```python
from build123d import *

# Parameters (mm, degrees)
BOSS_EXTRUDE1_DEPTH          = 6
FILLET1_R                    = 20
SKETCH2_R                    = 1.7
CUT_EXTRUDE1_DEPTH           = 133.106886392
CIRPATTERN1_COUNT            = 4
SKETCH3_R                    = 1.6
CUT_EXTRUDE2_DEPTH           = 133.106886392
LPATTERN1_COUNT              = 6
LPATTERN1_PITCH              = 10
CIRPATTERN2_COUNT            = 4
CIRPATTERN2_COPY_1_SKETCH_R  = 1.6
CIRPATTERN2_COPY_1_DEPTH     = 133.106886392
CIRPATTERN2_COPY_2_SKETCH_R  = 1.6
CIRPATTERN2_COPY_2_DEPTH     = 133.106886392
CIRPATTERN2_COPY_3_SKETCH_R  = 1.6
CIRPATTERN2_COPY_3_DEPTH     = 133.106886392
CIRPATTERN2_COPY_4_SKETCH_R  = 1.6
CIRPATTERN2_COPY_4_DEPTH     = 133.106886392
CIRPATTERN2_COPY_5_SKETCH_R  = 1.6
CIRPATTERN2_COPY_5_DEPTH     = 133.106886392
CIRPATTERN2_COPY_6_SKETCH_R  = 1.6
CIRPATTERN2_COPY_6_DEPTH     = 133.106886392
CIRPATTERN2_COPY_7_SKETCH_R  = 1.6
CIRPATTERN2_COPY_7_DEPTH     = 133.106886392
CIRPATTERN2_COPY_8_SKETCH_R  = 1.6
CIRPATTERN2_COPY_8_DEPTH     = 133.106886392
CIRPATTERN2_COPY_9_SKETCH_R  = 1.6
CIRPATTERN2_COPY_9_DEPTH     = 133.106886392
CIRPATTERN2_COPY_10_SKETCH_R = 1.6
CIRPATTERN2_COPY_10_DEPTH    = 133.106886392
CIRPATTERN2_COPY_11_SKETCH_R = 1.6
CIRPATTERN2_COPY_11_DEPTH    = 133.106886392
CIRPATTERN2_COPY_12_SKETCH_R = 1.6
CIRPATTERN2_COPY_12_DEPTH    = 133.106886392
CIRPATTERN2_COPY_13_SKETCH_R = 1.6
CIRPATTERN2_COPY_13_DEPTH    = 133.106886392
CIRPATTERN2_COPY_14_SKETCH_R = 1.6
CIRPATTERN2_COPY_14_DEPTH    = 133.106886392
CIRPATTERN2_COPY_15_SKETCH_R = 1.6
CIRPATTERN2_COPY_15_DEPTH    = 133.106886392
SKETCH4_R                    = 1.7
CUT_EXTRUDE3_DEPTH           = 133.106886392
CIRPATTERN3_COUNT            = 4
SKETCH5_R                    = 1.7
CUT_EXTRUDE4_DEPTH           = 133.106886392
SKETCH7_R                    = 1.7
CUT_EXTRUDE5_DEPTH           = 133.106886392
LPATTERN2_COUNT              = 2
LPATTERN2_PITCH              = 10
LPATTERN2_COL_COUNT          = 2
LPATTERN2_COL_PITCH          = 10
MIRROR2_COPY_1_SKETCH_R      = 1.7
MIRROR2_COPY_1_DEPTH         = 133.106886392
MIRROR2_COPY_2_SKETCH_R      = 1.7
MIRROR2_COPY_2_DEPTH         = 133.106886392


with BuildPart() as part:
    # Sketch1 → Boss-Extrude1 (new body)
    with BuildSketch(Plane(origin=(0, 0, 0), x_dir=(1, 0, 0), z_dir=(0, 1, 0))):
        with BuildLine():
            Line((-72.831998462, 89.802561211), (-13.029437252, 30))
            Line((-13.029437252, 30), (13.029437252, 30))
            Line((13.029437252, 30), (72.831998462, 89.802561211))
            ThreePointArc((72.831998462, 89.802561211), (89.802561211, 89.802561211), (89.802561211, 72.831998462))
            Line((89.802561211, 72.831998462), (30, 13.029437252))
            Line((30, 13.029437252), (30, -13.029437252))
            Line((30, -13.029437252), (89.802561211, -72.831998462))
            ThreePointArc((89.802561211, -72.831998462), (89.802561211, -89.802561211), (72.831998462, -89.802561211))
            Line((72.831998462, -89.802561211), (13.029437252, -30))
            Line((13.029437252, -30), (-13.029437252, -30))
            Line((-13.029437252, -30), (-72.831998462, -89.802561211))
            ThreePointArc((-72.831998462, -89.802561211), (-89.802561211, -89.802561211), (-89.802561211, -72.831998462))
            Line((-89.802561211, -72.831998462), (-30, -13.029437252))
            Line((-30, -13.029437252), (-30, 13.029437252))
            Line((-30, 13.029437252), (-89.802561211, 72.831998462))
            ThreePointArc((-89.802561211, 72.831998462), (-89.802561211, 89.802561211), (-72.831998462, 89.802561211))
        make_face()
    extrude(amount=BOSS_EXTRUDE1_DEPTH)

    # Fillet1
    fillet1_edges = [part.edges().sort_by_distance(p)[0] for p in [
        (-13.029437252, 3, -30),
        (13.029437252, 3, -30),
        (30, 3, -13.029437252),
        (30, 3, 13.029437252),
        (13.029437252, 3, 30),
        (-13.029437252, 3, 30),
        (-30, 3, 13.029437252),
        (-30, 3, -13.029437252),
    ]]
    fillet(fillet1_edges, radius=FILLET1_R)

    # Sketch2 → Cut-Extrude1 (cut, through all)
    with BuildSketch(Plane(origin=(0, 6, 0), x_dir=(1, 0, 0), z_dir=(0, 1, 0))):
        with Locations(Location((-22.525, -22.525, 0), (0, 0, 270))):
            Circle(SKETCH2_R)
    cut_extrude1 = extrude(amount=-CUT_EXTRUDE1_DEPTH, mode=Mode.SUBTRACT)

    # CirPattern1: Cut-Extrude1 ×4 about axis
    cirpattern1_axis = Axis((0, 0, 0), (0, 1, 0))
    for i in range(1, CIRPATTERN1_COUNT):
        add(cut_extrude1.rotate(cirpattern1_axis, i * 360 / CIRPATTERN1_COUNT), mode=Mode.SUBTRACT)

    # Sketch3 → Cut-Extrude2 (cut, through all)
    with BuildSketch(Plane(origin=(0, 6, 0), x_dir=(1, 0, 0), z_dir=(0, 1, 0))):
        with Locations(Location((-30, -30, 0), (0, 0, 270))):
            Circle(SKETCH3_R)
    cut_extrude2 = extrude(amount=-CUT_EXTRUDE2_DEPTH, mode=Mode.SUBTRACT)

    # LPattern1: Cut-Extrude2 ×6
    with Locations(*[Vector(-0.7071067811865467, 0, 0.7071067811865485) * (i * LPATTERN1_PITCH) for i in range(1, LPATTERN1_COUNT)]):
        add(cut_extrude2, mode=Mode.SUBTRACT)

    # CirPattern2: Cut-Extrude2 ×4 about axis
    cirpattern2_axis = Axis((0, 6.3, 0), (0, -1, 0))
    for i in range(1, CIRPATTERN2_COUNT):
        add(cut_extrude2.rotate(cirpattern2_axis, i * 360 / CIRPATTERN2_COUNT), mode=Mode.SUBTRACT)

    # CirPattern2 copy 1 sketch → CirPattern2 copy 1 (cut, through all)
    with BuildSketch(Plane(origin=(-7.071067812, 6, -7.071067812), x_dir=(0, 0, 1), z_dir=(0, 1, 0))):
        with Locations(Location((-30, -30, 0), (0, 0, 270))):
            Circle(CIRPATTERN2_COPY_1_SKETCH_R)
    extrude(amount=-CIRPATTERN2_COPY_1_DEPTH, mode=Mode.SUBTRACT)

    # CirPattern2 copy 2 sketch → CirPattern2 copy 2 (cut, through all)
    with BuildSketch(Plane(origin=(7.071067812, 6, -7.071067812), x_dir=(-1, 0, 0), z_dir=(0, 1, 0))):
        with Locations(Location((-30, -30, 0), (0, 0, 270))):
            Circle(CIRPATTERN2_COPY_2_SKETCH_R)
    extrude(amount=-CIRPATTERN2_COPY_2_DEPTH, mode=Mode.SUBTRACT)

    # CirPattern2 copy 3 sketch → CirPattern2 copy 3 (cut, through all)
    with BuildSketch(Plane(origin=(7.071067812, 6, 7.071067812), x_dir=(0, 0, -1), z_dir=(0, 1, 0))):
        with Locations(Location((-30, -30, 0), (0, 0, 270))):
            Circle(CIRPATTERN2_COPY_3_SKETCH_R)
    extrude(amount=-CIRPATTERN2_COPY_3_DEPTH, mode=Mode.SUBTRACT)

    # CirPattern2 copy 4 sketch → CirPattern2 copy 4 (cut, through all)
    with BuildSketch(Plane(origin=(-14.142135624, 6, -14.142135624), x_dir=(0, 0, 1), z_dir=(0, 1, 0))):
        with Locations(Location((-30, -30, 0), (0, 0, 270))):
            Circle(CIRPATTERN2_COPY_4_SKETCH_R)
    extrude(amount=-CIRPATTERN2_COPY_4_DEPTH, mode=Mode.SUBTRACT)

    # CirPattern2 copy 5 sketch → CirPattern2 copy 5 (cut, through all)
    with BuildSketch(Plane(origin=(14.142135624, 6, -14.142135624), x_dir=(-1, 0, 0), z_dir=(0, 1, 0))):
        with Locations(Location((-30, -30, 0), (0, 0, 270))):
            Circle(CIRPATTERN2_COPY_5_SKETCH_R)
    extrude(amount=-CIRPATTERN2_COPY_5_DEPTH, mode=Mode.SUBTRACT)

    # CirPattern2 copy 6 sketch → CirPattern2 copy 6 (cut, through all)
    with BuildSketch(Plane(origin=(14.142135624, 6, 14.142135624), x_dir=(0, 0, -1), z_dir=(0, 1, 0))):
        with Locations(Location((-30, -30, 0), (0, 0, 270))):
            Circle(CIRPATTERN2_COPY_6_SKETCH_R)
    extrude(amount=-CIRPATTERN2_COPY_6_DEPTH, mode=Mode.SUBTRACT)

    # CirPattern2 copy 7 sketch → CirPattern2 copy 7 (cut, through all)
    with BuildSketch(Plane(origin=(-21.213203436, 6, -21.213203436), x_dir=(0, 0, 1), z_dir=(0, 1, 0))):
        with Locations(Location((-30, -30, 0), (0, 0, 270))):
            Circle(CIRPATTERN2_COPY_7_SKETCH_R)
    extrude(amount=-CIRPATTERN2_COPY_7_DEPTH, mode=Mode.SUBTRACT)

    # CirPattern2 copy 8 sketch → CirPattern2 copy 8 (cut, through all)
    with BuildSketch(Plane(origin=(21.213203436, 6, -21.213203436), x_dir=(-1, 0, 0), z_dir=(0, 1, 0))):
        with Locations(Location((-30, -30, 0), (0, 0, 270))):
            Circle(CIRPATTERN2_COPY_8_SKETCH_R)
    extrude(amount=-CIRPATTERN2_COPY_8_DEPTH, mode=Mode.SUBTRACT)

    # CirPattern2 copy 9 sketch → CirPattern2 copy 9 (cut, through all)
    with BuildSketch(Plane(origin=(21.213203436, 6, 21.213203436), x_dir=(0, 0, -1), z_dir=(0, 1, 0))):
        with Locations(Location((-30, -30, 0), (0, 0, 270))):
            Circle(CIRPATTERN2_COPY_9_SKETCH_R)
    extrude(amount=-CIRPATTERN2_COPY_9_DEPTH, mode=Mode.SUBTRACT)

    # CirPattern2 copy 10 sketch → CirPattern2 copy 10 (cut, through all)
    with BuildSketch(Plane(origin=(-28.284271247, 6, -28.284271247), x_dir=(0, 0, 1), z_dir=(0, 1, 0))):
        with Locations(Location((-30, -30, 0), (0, 0, 270))):
            Circle(CIRPATTERN2_COPY_10_SKETCH_R)
    extrude(amount=-CIRPATTERN2_COPY_10_DEPTH, mode=Mode.SUBTRACT)

    # CirPattern2 copy 11 sketch → CirPattern2 copy 11 (cut, through all)
    with BuildSketch(Plane(origin=(28.284271247, 6, -28.284271247), x_dir=(-1, 0, 0), z_dir=(0, 1, 0))):
        with Locations(Location((-30, -30, 0), (0, 0, 270))):
            Circle(CIRPATTERN2_COPY_11_SKETCH_R)
    extrude(amount=-CIRPATTERN2_COPY_11_DEPTH, mode=Mode.SUBTRACT)

    # CirPattern2 copy 12 sketch → CirPattern2 copy 12 (cut, through all)
    with BuildSketch(Plane(origin=(28.284271247, 6, 28.284271247), x_dir=(0, 0, -1), z_dir=(0, 1, 0))):
        with Locations(Location((-30, -30, 0), (0, 0, 270))):
            Circle(CIRPATTERN2_COPY_12_SKETCH_R)
    extrude(amount=-CIRPATTERN2_COPY_12_DEPTH, mode=Mode.SUBTRACT)

    # CirPattern2 copy 13 sketch → CirPattern2 copy 13 (cut, through all)
    with BuildSketch(Plane(origin=(-35.355339059, 6, -35.355339059), x_dir=(0, 0, 1), z_dir=(0, 1, 0))):
        with Locations(Location((-30, -30, 0), (0, 0, 270))):
            Circle(CIRPATTERN2_COPY_13_SKETCH_R)
    extrude(amount=-CIRPATTERN2_COPY_13_DEPTH, mode=Mode.SUBTRACT)

    # CirPattern2 copy 14 sketch → CirPattern2 copy 14 (cut, through all)
    with BuildSketch(Plane(origin=(35.355339059, 6, -35.355339059), x_dir=(-1, 0, 0), z_dir=(0, 1, 0))):
        with Locations(Location((-30, -30, 0), (0, 0, 270))):
            Circle(CIRPATTERN2_COPY_14_SKETCH_R)
    extrude(amount=-CIRPATTERN2_COPY_14_DEPTH, mode=Mode.SUBTRACT)

    # CirPattern2 copy 15 sketch → CirPattern2 copy 15 (cut, through all)
    with BuildSketch(Plane(origin=(35.355339059, 6, 35.355339059), x_dir=(0, 0, -1), z_dir=(0, 1, 0))):
        with Locations(Location((-30, -30, 0), (0, 0, 270))):
            Circle(CIRPATTERN2_COPY_15_SKETCH_R)
    extrude(amount=-CIRPATTERN2_COPY_15_DEPTH, mode=Mode.SUBTRACT)

    # Sketch4 → Cut-Extrude3 (cut, through all)
    with BuildSketch(Plane(origin=(0, 6, 0), x_dir=(1, 0, 0), z_dir=(0, 1, 0))):
        with Locations(Location((-86.974134086, -86.974134086, 0), (0, 0, 270))):
            Circle(SKETCH4_R)
        with Locations(Location((-86.974134086, -75.660425587, 0), (0, 0, 270))):
            Circle(SKETCH4_R)
        with Locations(Location((-75.660425587, -75.660425587, 0), (0, 0, 270))):
            Circle(SKETCH4_R)
        with Locations(Location((-75.660425587, -86.974134086, 0), (0, 0, 270))):
            Circle(SKETCH4_R)
    cut_extrude3 = extrude(amount=-CUT_EXTRUDE3_DEPTH, mode=Mode.SUBTRACT)

    # CirPattern3: Cut-Extrude3 ×4 about axis
    cirpattern3_axis = Axis((0, 0, 0), (0, 1, 0))
    for i in range(1, CIRPATTERN3_COUNT):
        add(cut_extrude3.rotate(cirpattern3_axis, i * 360 / CIRPATTERN3_COUNT), mode=Mode.SUBTRACT)

    # Sketch5 → Cut-Extrude4 (cut, through all)
    with BuildSketch(Plane(origin=(0, 6, 0), x_dir=(1, 0, 0), z_dir=(0, 1, 0))):
        with Locations(Location((-22.525, 27.375, 0), (0, 0, 270))):
            Circle(SKETCH5_R)
        with Locations(Location((-22.525, -27.35, 0), (0, 0, 270))):
            Circle(SKETCH5_R)
    cut_extrude4 = extrude(amount=-CUT_EXTRUDE4_DEPTH, mode=Mode.SUBTRACT)

    # Mirror1: Cut-Extrude4 across plane
    add(cut_extrude4.mirror(Plane(origin=(0, 0, 0), x_dir=(0, 0, 1), z_dir=(1, 0, 0))), mode=Mode.SUBTRACT)

    # Sketch7 → Cut-Extrude5 (cut, through all)
    with BuildSketch(Plane(origin=(0, 6, 0), x_dir=(1, 0, 0), z_dir=(0, 1, 0))):
        with Locations(Location((-27, 0, 0), (0, 0, 270))):
            Circle(SKETCH7_R)
    cut_extrude5 = extrude(amount=-CUT_EXTRUDE5_DEPTH, mode=Mode.SUBTRACT)

    # LPattern2: Cut-Extrude5 ×2
    with Locations(*[(0, 0, i * LPATTERN2_PITCH) for i in range(1, LPATTERN2_COUNT)]):
        add(cut_extrude5, mode=Mode.SUBTRACT)

    # LPattern2 col: Cut-Extrude5 ×2
    with Locations(*[(0, 0, -i * LPATTERN2_COL_PITCH) for i in range(1, LPATTERN2_COL_COUNT)]):
        add(cut_extrude5, mode=Mode.SUBTRACT)

    # Mirror2: Cut-Extrude5 across plane
    add(cut_extrude5.mirror(Plane(origin=(0, 0, 0), x_dir=(0, 0, 1), z_dir=(1, 0, 0))), mode=Mode.SUBTRACT)

    # Mirror2 copy 1 sketch → Mirror2 copy 1 (cut, through all)
    with BuildSketch(Plane(origin=(0, 6, 10), x_dir=(-1, 0, 0), z_dir=(0, 1, 0))):
        with Locations((-27, 0)):
            Circle(MIRROR2_COPY_1_SKETCH_R)
    extrude(amount=-MIRROR2_COPY_1_DEPTH, mode=Mode.SUBTRACT)

    # Mirror2 copy 2 sketch → Mirror2 copy 2 (cut, through all)
    with BuildSketch(Plane(origin=(0, 6, -10), x_dir=(-1, 0, 0), z_dir=(0, 1, 0))):
        with Locations((-27, 0)):
            Circle(MIRROR2_COPY_2_SKETCH_R)
    extrude(amount=-MIRROR2_COPY_2_DEPTH, mode=Mode.SUBTRACT)


solid = part.part
```
Part model, mm, in its own coordinate system. A direction names the side the tool comes from. Coordinates: 2 decimals unless noted, no trailing zeros. Order: outer loops, then holes, each group sorted by start corner. A loop starts at its lowest first (then second) coordinate and runs counter-clockwise, first axis right, second up. Notation, with made-up numbers: (52.5, 2) -> (88.5, 2) arc R25 ccw to (88.5, 25) -> close; hole circle Ø4 at (0.25, 40.5). An arc over 180 degrees is marked (long way). Put each result on its own line as item: value. Start each with the question number.
(1) Which spindle directions (+Z, -Z, +X, -X, +Y, -Y) get a long thin tool onto all of the face, cutting with end or side? Do faces 1 (the face through (-89.6, 3, 90)), 2 (the face through (12.5, 3.042, 31.565)), 3 (the face through (30, 3, 0)), 4 (the face through (-30, 3, 0)), 5 (the face through (-12.5, 3.042, -31.565)). Say none if no direction does.
(2) Probe line 1 along Z through (x, y) = (-66, 5.45); line 2 along Z through (x, y) = (74.5, 1.8); line 3 along Z through (x, y) = (23, 1.45). List the from-to ranges inside material, lowest first. Write a range as [from, to].
(3) Pin check, flat tips, straight feed: pin 1 Ø1.5 at (x, y) = (62, 3.5) entering from -Z; pin 2 Ø1.8 at (x, y) = (1.5, 3.5) entering from -Z; pin 3 Ø3 at (y, z) = (1, 54.5) entering from -X. Stop position of each tip, or through.
(4) Band-saw the part on B-B (y = 1). Count the separate pieces of the cut face and the enclosed holes in it, then the cut area to 3 significant figures.
(5) Band-saw the part on A-A (x = -9). Give the cut face in (y, z), then the cut area to 3 significant figures.
(6) Mould opens along Z. For faces 6 (the face through (-31.565, 3.042, 12.5)), 7 (the face through (0, 3, 30)), 8 (the face through (-90, 3, -89.6)), 9 (the face through (45.48, 2.96, -62.45)) say: pulls with the +Z half, pulls with the -Z half, needs draft (parallel to the pull), parting line crosses it, or undercut.
Determined:
1. face 1: +Y, -Y
1. face 2: +Z, +Y, -Y
1. face 3: +X, +Y, -Y
1. face 4: -X, +Y, -Y
1. face 5: -Z, +Y, -Y
2. line 1: z = [-82.97, -66.82], [-63.89, -49.03], [49.03, 63.89], [66.82, 82.97]
2. line 2: z = [-91.19, -88.22], [-85.73, -76.9], [-74.42, -57.53], [57.53, 74.42], [76.9, 85.73], [88.22, 91.19]
2. line 3: z = [-39.97, -29.01], [-25.74, -24.16], [-20.89, 20.89], [24.16, 25.72], [28.98, 39.97]
3. pin 1: stops at z = -79.72
3. pin 2: stops at z = -30
3. pin 3: stops at x = -72.97
4. separate pieces: 1
4. enclosed holes: 54
4. area: 11,700 mm²
5. outline: (0, -30.46) -> (6, -30.46) -> (6, 30.46) -> (0, 30.46) -> close
5. area: 365 mm²
6. face 6: undercut
6. face 7: pulls with the +Z half
6. face 8: undercut
6. face 9: pulls with the -Z half
